```python
from build123d import *

# Parameters (mm, degrees)
SKETCH1_W           = 222.25
SKETCH1_H           = 95.25
BOSS_EXTRUDE1_DEPTH = 5.08
SKETCH2_W           = 218.44
SKETCH2_H           = 2.54
CUT_EXTRUDE1_DEPTH  = 5.08
SKETCH5_W           = 2.54
SKETCH5_H           = 15.24
CUT_EXTRUDE4_DEPTH  = 5.08
SKETCH7_W           = 28.575
SKETCH7_H           = 21.74875
CUT_EXTRUDE5_DEPTH  = 5.08
SKETCH8_W           = 28.575
SKETCH8_H           = 21.2725
CUT_EXTRUDE6_DEPTH  = 5.08
SKETCH11_W          = 28.575
SKETCH11_H          = 10.16
CUT_EXTRUDE8_DEPTH  = 5.08
BOSS_EXTRUDE2_DEPTH = 58.42
SKETCH12_W          = 12.7
SKETCH12_H          = 50.8
CUT_EXTRUDE9_DEPTH  = 2.54


with BuildPart() as part:
    # Sketch1 → Boss-Extrude1 (new body)
    with BuildSketch(Plane.XY):
        Rectangle(SKETCH1_W, SKETCH1_H)
    extrude(amount=BOSS_EXTRUDE1_DEPTH)

    # Sketch2 → Cut-Extrude1 (cut)
    with BuildSketch(Plane(origin=(0, 0, 0), x_dir=(-1, 0, 0), z_dir=(0, 0, -1))):
        with Locations((0, 24.60625)):
            Rectangle(SKETCH2_W, SKETCH2_H)
        with Locations((0, 11.90625)):
            Rectangle(SKETCH2_W, SKETCH2_H)
        with Locations((0, 37.30625)):
            Rectangle(SKETCH2_W, SKETCH2_H)
        with Locations((0, -11.90625)):
            Rectangle(SKETCH2_W, SKETCH2_H)
        with Locations((0, -24.60625)):
            Rectangle(SKETCH2_W, SKETCH2_H)
        with Locations((0, -37.30625)):
            Rectangle(SKETCH2_W, SKETCH2_H)
    extrude(amount=-CUT_EXTRUDE1_DEPTH, mode=Mode.SUBTRACT)

    # Sketch5 → Cut-Extrude4 (cut)
    with BuildSketch(Plane(origin=(0, 0, 0), x_dir=(-1, 0, 0), z_dir=(0, 0, -1))):
        with Locations((-85.725, 0)):
            Rectangle(SKETCH5_W, SKETCH5_H)
    extrude(amount=-CUT_EXTRUDE4_DEPTH, mode=Mode.SUBTRACT)

    # Sketch7 → Cut-Extrude5 (cut)
    with BuildSketch(Plane(origin=(0, 0, 0), x_dir=(-1, 0, 0), z_dir=(0, 0, -1))):
        with Locations((-20.6375, 36.750625)):
            Rectangle(SKETCH7_W, SKETCH7_H)
    extrude(amount=-CUT_EXTRUDE5_DEPTH, mode=Mode.SUBTRACT)

    # Sketch8 → Cut-Extrude6 (cut)
    with BuildSketch(Plane(origin=(0, 0, 0), x_dir=(-1, 0, 0), z_dir=(0, 0, -1))):
        with Locations((-20.6375, 0)):
            Rectangle(SKETCH8_W, SKETCH8_H)
    extrude(amount=-CUT_EXTRUDE6_DEPTH, mode=Mode.SUBTRACT)

    # Sketch11 → Cut-Extrude8 (cut)
    with BuildSketch(Plane(origin=(0, 0, 0), x_dir=(-1, 0, 0), z_dir=(0, 0, -1))):
        with Locations((-20.6375, 18.25625)):
            Rectangle(SKETCH11_W, SKETCH11_H)
    extrude(amount=-CUT_EXTRUDE8_DEPTH, mode=Mode.SUBTRACT)

    # Sketch10 → Boss-Extrude2 (add)
    with BuildSketch(Plane(origin=(0, 47.625, 0), x_dir=(1, 0, 0), z_dir=(0, 1, 0))):
        Polygon((6.35, 0), (6.35, 6.35), (26.67, 6.35), (34.925, -5.08), (34.925, 0), (29.21, 8.89), (3.81, 8.89), (3.81, 0), align=None)
    extrude(amount=-BOSS_EXTRUDE2_DEPTH)

    # Sketch12 → Cut-Extrude9 (cut)
    with BuildSketch(Plane.XY.offset(-6.35)):
        with Locations((16.51, 18.415)):
            Rectangle(SKETCH12_W, SKETCH12_H)
    extrude(amount=-CUT_EXTRUDE9_DEPTH, mode=Mode.SUBTRACT)


solid = part.part
```
Source: CAD feature listing. Evaluate the final solid. Frame: model axes, mm. A direction names the side the tool comes from. Coordinates: 2 decimals unless noted, no trailing zeros. Write each loop counter-clockwise with the first axis right and the second up, starting at its lowest first coordinate (ties: lowest second). Pieces come first, ordered by that corner, then holes. Notation, with made-up numbers: (-25.5, 43) -> (-16.5, 43) arc R28 ccw to (-16.5, 61) -> close; hole circle Ø2 at (-38.75, -16.75). An arc over 180 degrees is marked (long way). Return JSON: item names as keys, results as strings. Group by question number.
1) Mould query, pull axis Y, two halves, no side actions, for faces 4 (the face through (111.125, -1, 3)), 5 (the face through (-1, 47.625, 2)), 6 (the face through (73, 25.876, 3)), 7 (the face through (-2, -47.625, 3)). Classes: +Y half, -Y half, draft (parallel to the pull), parting line (faces both ways), or undercut.
2) Section query B-B, the plane x = 95.5. Return loops of the section in (y, z) (3 decimals).
3) Contact query for flat-ended pins moving along their axis: P1, Ø8, axis at x = 70.5, y = -28, coming from the -Z side; P2, Ø2, axis at y = 22.5, z = -7, coming from the +X side; P3, Ø1.5, axis at x = 23.5, z = 3, coming from the +Y side. Output: stop coordinate, or through.
4) Section query A-A, the plane y = 2.5. Return loops of the section in (x, z) (3 decimals), plus the area to 3 significant figures.
5) Ray query, line 1 along Y through (x, z) = (21.5, 3.25) (3 decimals); line 2 along Y through (x, z) = (25.5, -6.5) (3 decimals); line 3 along X through (y, z) = (21.5, 4.5) (3 decimals). Return the intervals inside material, ascending.
6) Set-up query: faces 1 (the face through (73, -10.636, 3)), 2 (the face through (23.1, 18.8, -6.35)), 3 (the face through (30.74, 18.824, -0.715)). Return all of +Z, -Z, +X, -X, +Y, -Y with unobstructed straight access to the full face (end or side cutting, diameter ignored); none if empty.
7) Section query C-C, the plane z = -2. Return loops of the section in (x, y) (3 decimals), plus the area to 3 significant figures.
8) Section query D-D, the plane y = -16.5. Return loops of the section in (x, z) (3 decimals).
From the geometry:
{
 "1": {"face 4": "draft", "face 5": "+Y half", "face 6": "undercut", "face 7": "-Y half"},
 "2": {"outline": "(-47.625, 0) -> (-38.576, 0) -> (-38.576, 5.08) -> (-47.625, 5.08) -> close; (-36.036, 0) -> (-25.876, 0) -> (-25.876, 5.08) -> (-36.036, 5.08) -> close; (-23.336, 0) -> (-13.176, 0) -> (-13.176, 5.08) -> (-23.336, 5.08) -> close; (-10.636, 0) -> (10.636, 0) -> (10.636, 5.08) -> (-10.636, 5.08) -> close; (13.176, 0) -> (23.336, 0) -> (23.336, 5.08) -> (13.176, 5.08) -> close; (25.876, 0) -> (36.036, 0) -> (36.036, 5.08) -> (25.876, 5.08) -> close; (38.576, 0) -> (47.625, 0) -> (47.625, 5.08) -> (38.576, 5.08) -> close"},
 "3": {"P1": "z = 0", "P2": "x = 31.07", "P3": "y = -13.18"},
 "4": {"outline": "(-111.125, 0) -> (3.81, 0) -> (3.81, -8.89) -> (10.16, -8.89) -> (10.16, -6.35) -> (6.35, -6.35) -> (6.35, 5.08) -> (-111.125, 5.08) -> close; (22.86, -8.89) -> (29.21, -8.89) -> (34.925, 0) -> (84.455, 0) -> (84.455, 5.08) -> (34.925, 5.08) -> (26.67, -6.35) -> (22.86, -6.35) -> close; (86.995, 0) -> (111.125, 0) -> (111.125, 5.08) -> (86.995, 5.08) -> close", "area": "1,060 mm²"},
 "5": {"line 1": "-47.625 to -38.576, -36.036 to -25.876, -23.336 to -13.176", "line 2": "-10.795 to 47.625", "line 3": "-111.125 to 6.35, 34.506 to 111.125"},
 "6": {"face 1": "+Z, -Z", "face 2": "+Z, +Y, -Y", "face 3": "+Z, +Y"},
 "7": {"outline": "(3.81, -10.795) -> (6.35, -10.795) -> (6.35, 47.625) -> (3.81, 47.625) -> close; (29.812, -10.795) -> (33.639, -10.795) -> (33.639, 47.625) -> (29.812, 47.625) -> close", "area": "372 mm²"},
 "8": {"outline": "(-111.125, 0) -> (111.125, 0) -> (111.125, 5.08) -> (-111.125, 5.08) -> close"}
}
